Autodesk Inventor part; units mm, degrees
ref_plane "WorkPlane1" through (0, 0, 0) normal (0, 0, 1) x (1, 0, 0)
ref_plane "MSC_PF1" through (0, 0, 0) normal (1, 0, 0) x (0, 1, 0)
ref_plane "MSC_PT1" through (0, 0, 0) normal (0, 0, -1) x (-1, 0, 0)
ref_plane "WorkPlane1" through (0, 0, 0) normal (0, 0, 1) x (1, 0, 0)
sketch "Sketch1" plane through (0, 0, 0) normal (0, 0, 1) x (1, 0, 0)
  point P0 (0, 0)
sketch "Sketch2" plane through (0, 0, 0) normal (0, 0, 1) x (1, 0, 0)
  line L0 (-5, 2.8868) -> (-5, -2.8868)
  line L1 (0, 5.7734) -> (-5, 2.8868)
  line L2 (5, 2.8868) -> (0, 5.7734)
  line L3 (5, -2.8868) -> (5, 2.8868)
  line L4 (0, -5.7734) -> (5, -2.8868)
  line L5 (-5, -2.8868) -> (0, -5.7734)
  circle A0 centre (0, 0) radius 5 construction
  dimension "d1" = 10
  dimension "d29" = 0
  dimension "d30" = 0
extrude "Extrusion1" add sketch "Sketch2" along normal blind 4
sketch "Sketch3" plane through (0, 0, 0) normal (1, 0, 0) x (0, 1, 0)
  line L0 (5, 4) -> (5.8734, 4)
  line L1 (5.8734, 3.4957) -> (5, 4)
  line L2 (5.8734, 4) -> (5.8734, 3.4957)
  line L3 (0, -0.8) -> (0, 4.8)
  line L4 (5.7734, 0) -> (5.7734, 4)
  dimension "d25" = 0.1
  dimension "d26" = 0
  dimension "d27" = 60
  dimension "d28" = 5
revolve "Revolution1" cut sketch "Sketch3" angle 360 about axis through (0, 0, -10) along (0, 0, 1)
sketch "Sketch4" plane through (0, 0, 0) normal (1, 0, 0) x (0, 1, 0)
  line L0 (0, -60) -> (0, 0)
  line L1 (-3, -60) -> (0, -60)
  line L2 (-3, 0) -> (-3, -60)
  line L3 (0, 0) -> (-3, 0)
  line L4 (0, -60) -> (0, 0)
  line L5 (-3.6, 0) -> (0.6, 0)
  line L6 (0, -72) -> (0, 12)
  dimension "d18" = 3
  dimension "d20" = 60
  dimension "d33" = 0
  dimension "d34" = 0
revolve "Revolution2" add sketch "Sketch4" angle 360 about axis through (0, 0, -60) along (0, 0, -1)
chamfer "Chamfer1" distance 0.5 angle 45 1 edges at (0, 3, -60)
fillet "Fillet1" radius 0.25 1 edges at (0, 3, 0)
thread "Thread1"
ref_plane "MSC_PF1" through (0, 0, 0) normal (1, 0, 0) x (0, 1, 0)
ref_plane "MSC_PT1" through (0, 0, 0) normal (0, 0, -1) x (-1, 0, 0)
equation "\"d22\" = 0.5 * PTC"
equation "\"d23\" = 0.5 * PTC"
equation "\"d24\" = r"
equation "\"d1\" = ParS"
equation "\"d6\" = ParK"
equation "\"b\" = NLG - 2 * PTC"
equation "\"d28\" = 0.5 * ParS"
equation "\"d18\" = 0.5 * NND"
equation "\"d20\" = NLG"
equation "\"NND\" = 6"
equation "\"NLG\" = 60"
equation "\"PTC\" = 1"
equation "\"ParK\" = 4"
equation "\"ParS\" = 10"
equation "\"msp_es\" = 0.577367 * ParS"
equation "\"r\" = 0.25"
equation "\"THREADDIA\" = NND"
properties part number "ISO 4018 - M6 x 60" material "Steel"
Geometry check sheet. Reference: the model listing, model coordinates, mm. Give positions to 0.01 mm unless a question says otherwise; leave off trailing zeros. Write each loop counter-clockwise with the first axis right and the second up, starting at its lowest first coordinate (ties: lowest second). Pieces come first, ordered by that corner, then holes. Notation, with made-up numbers: (16.25, 27) -> (55.25, 27) arc R15 cw to (55.25, 50) -> close; hole circle Ø5 at (67, 80.5). An arc over 180 degrees is marked (long way). One line per question, with ' | ' between items.
Item 1: Draft check along X on faces 1 (the flat face through (2.535, 4.31, 1.972)), 2 (the cylindrical face through (0, 3, -30)), 3 (the flat face through (-3.4, 0.1, 0)), 4 (the conical face through (-4.515, -2.612, 3.875)). Enter one of: released by +X, released by -X, zero draft, split by the parting line, or undercut.
Determined:
face 1: released by +X | face 2: split by the parting line | face 3: zero draft | face 4: released by -X
Item 2: Scan lines: line 1 along X through (y, z) = (0, -55); line 2 along Z through (x, y) = (-3.5, 2.25); line 3 along X through (y, z) = (-2, -41.5). Record each from-to range of solid material in increasing order.
Determined:
line 1: -3 to 3 | line 2: 0 to 4 | line 3: -2.24 to 2.24
Item 3: Depth check by flat-ended pin: pin 1 (3 mm diameter, centred on x = 1, z = -42, fed in from -Y); pin 2 (3 mm diameter, centred on x = -3.5, z = -26, fed in from -Y); pin 3 (1.5 mm diameter, centred on x = -1.5, z = -37.5, fed in from +Y). Enter the tip coordinate at first touch or a pass-through.
Determined:
pin 1: y = -3 | pin 2: y = -2.24 | pin 3: y = 2.9
Item 4: Sectioned sample at A-A, the plane z = -26.5. Record the boundary of the cut face in (x, y), plus the area to 3 significant figures.
Determined:
outline: circle Ø6 at (0, 0) | area: 28.3 mm^2
